Input: part model. Units: mm. Frame: model coordinates. A direction names the side the tool comes from. Coordinates: 2 decimals unless noted, no trailing zeros. Loops run counter-clockwise (first coordinate to the right, second up) from the corner with the lowest first, then second, coordinate; pieces in that order, holes last.
(1) Set-up query: faces 4 (the face through (-6.1, 0, -184.734)), 5 (the face through (-6.345, -0.257, -46.414)). Return all of +Z, -Z, +X, -X, +Y, -Y with unobstructed straight access to the full face (end or side cutting, diameter ignored); none if empty.
(2) Section B-B, the plane y = -3.75. Return loops of the section in (x, z), then the cut area to 3 significant figures.
(3) Contact query for flat-ended pins moving along their axis: P1, Ø1, axis at y = -1, z = -34, coming from the -X side; P2, Ø1.5, axis at x = 6, z = -77, coming from the -Y side; P3, Ø6, axis at y = 2.5, z = -120.5, coming from the +X side. Output: stop coordinate, or through.
(4) Section A-A, the plane x = 2.25. Return loops of the section in (y, z).
(5) Mould query, pull axis Z, two halves, no side actions, for faces 1 (the face through (-6.345, 0.257, -194.34)), 2 (the face through (-5.94, 0.24, 96.34)), 3 (the face through (0, 0, -203.2)). Classes: released by +Z, released by -Z, zero draft, split by the parting line, or undercut.
(6) Section C-C, the plane z = -42. Return loops of the section in (x, y).
(7) Line query: L1, parallel to Z at x = -4, y = -4.5; L2, parallel to Y at x = 0.75, z = -62.5; L3, parallel to Y at x = 5, z = -137. Output: solid intervals per line, ascending.
Autodesk Inventor part; units mm, degrees
sketch "Sketch1" plane through (0, 0, 0) normal (0, 0, 1) x (1, 0, 0)
  circle A0 centre (0, 0) radius 6.35
  dimension "d0" = 12.7
extrude "Extrusion1" add sketch "Sketch1" along normal mid plane 406.4
ref_plane "Work Plane1" through (0, 0, 203.2) normal (0, 0, 1) x (1, 0, 0)
ref_plane "Work Plane2" through (0, 0, -185.7248) normal (0, 0, -1) x (-1, 0, 0)
sketch "Sketch2" plane through (0, 0, -185.7248) normal (0, 0, -1) x (-1, 0, 0)
  circle A0 centre (0, 0) radius 5.9436
  circle A1 centre (0, 0) radius 6.35
  dimension "d5" = 11.8872
  dimension "d6" = 12.7
extrude "Extrusion2" cut sketch "Sketch2" against normal blind 0.9906
ref_plane "Work Plane3" through (0, 0, 96.8248) normal (0, 0, 1) x (1, 0, 0)
sketch "Sketch3" plane through (0, 0, 96.8248) normal (0, 0, 1) x (1, 0, 0)
  circle A0 centre (0, 0) radius 6.35
  circle A1 centre (0, 0) radius 5.9436
  dimension "d10" = 12.7
  dimension "d11" = 11.8872
extrude "Extrusion3" cut sketch "Sketch3" against normal blind 0.9906
ref_plane "Work Plane4" through (6.35, 0, 0) normal (1, 0, 0) x (0, 1, 0)
sketch "Sketch5" plane through (0, 0, -203.2) normal (0, 0, -1) x (-1, 0, 0)
  circle A0 centre (0, 0) radius 6.35
sketch "Sketch6" plane through (0, 0, -203.2) normal (0, 0, -1) x (-1, 0, 0)
  circle A0 centre (0, 0) radius 6.35
  line L0 (-4.7625, -1.5875) -> (-7.9375, -1.5875)
  line L1 (-7.9375, -1.5875) -> (-7.9375, 1.5875)
  line L2 (-7.9375, 1.5875) -> (-4.7625, 1.5875)
  line L3 (-4.7625, 1.5875) -> (-4.7625, -1.5875)
  line L4 (-4.7625, -1.5875) -> (-7.9375, 1.5875) construction
  line L5 (-7.9375, -1.5875) -> (-4.7625, 1.5875) construction
  point P0 (-6.35, 0)
  dimension "d19" = 3.175
  dimension "d20" = 3.175
extrude "Extrusion5" cut sketch "Sketch6" against normal blind 406.4 contours L2 L3 L0 A0 | A0 L0 L1 L2 picked at (-5.2842, -0.1781)
ref_plane "Midplane" through (0, 0, -44.45) normal (0, 0, 1) x (1, 0, 0)
sketch "Sketch7" plane through (0, 0, 203.2) normal (0, 0, 1) x (1, 0, 0)
  circle A0 centre (0, 0) radius 11.5682
extrude "Extrusion6" cut sketch "Sketch7" against normal blind 88.9
properties part number "Pin .5in. Dia. - Boom Hinge" material "Stainless Steel"
Report:
1. face 4: none
1. face 5: +Z, -Z
2. outline: (-5.12, -203.2) - (5.12, -203.2) - (5.12, -185.72) - (4.61, -185.72) - (4.61, -184.73) - (5.12, -184.73) - (5.12, 95.83) - (4.61, 95.83) - (4.61, 96.82) - (5.12, 96.82) - (5.12, 114.3) - (-5.12, 114.3) - (-5.12, 96.82) - (-4.61, 96.82) - (-4.61, 95.83) - (-5.12, 95.83) - (-5.12, -184.73) - (-4.61, -184.73) - (-4.61, -185.72) - (-5.12, -185.72) - close
2. area: 3,250 mm2
3. P1: stops at x = -6.33
3. P2: stops at y = -3.57
3. P3: stops at x = 6.15
4. outline: (-5.94, -203.2) - (5.94, -203.2) - (5.94, -185.72) - (5.5, -185.72) - (5.5, -184.73) - (5.94, -184.73) - (5.94, 95.83) - (5.5, 95.83) - (5.5, 96.82) - (5.94, 96.82) - (5.94, 114.3) - (-5.94, 114.3) - (-5.94, 96.82) - (-5.5, 96.82) - (-5.5, 95.83) - (-5.94, 95.83) - (-5.94, -184.73) - (-5.5, -184.73) - (-5.5, -185.72) - (-5.94, -185.72) - close
5. face 1: zero draft
5. face 2: undercut
5. face 3: released by -Z
6. outline: (4.76, -1.59) - (4.76, 1.59) - (6.15, 1.59) arc R6.35 ccw (long way) to (6.15, -1.59) - close
7. L1: z = -203.2 to -185.72, -184.73 to 95.83, 96.82 to 114.3
7. L2: y = -6.31 to 6.31
7. L3: y = -3.91 to -1.59, 1.59 to 3.91
